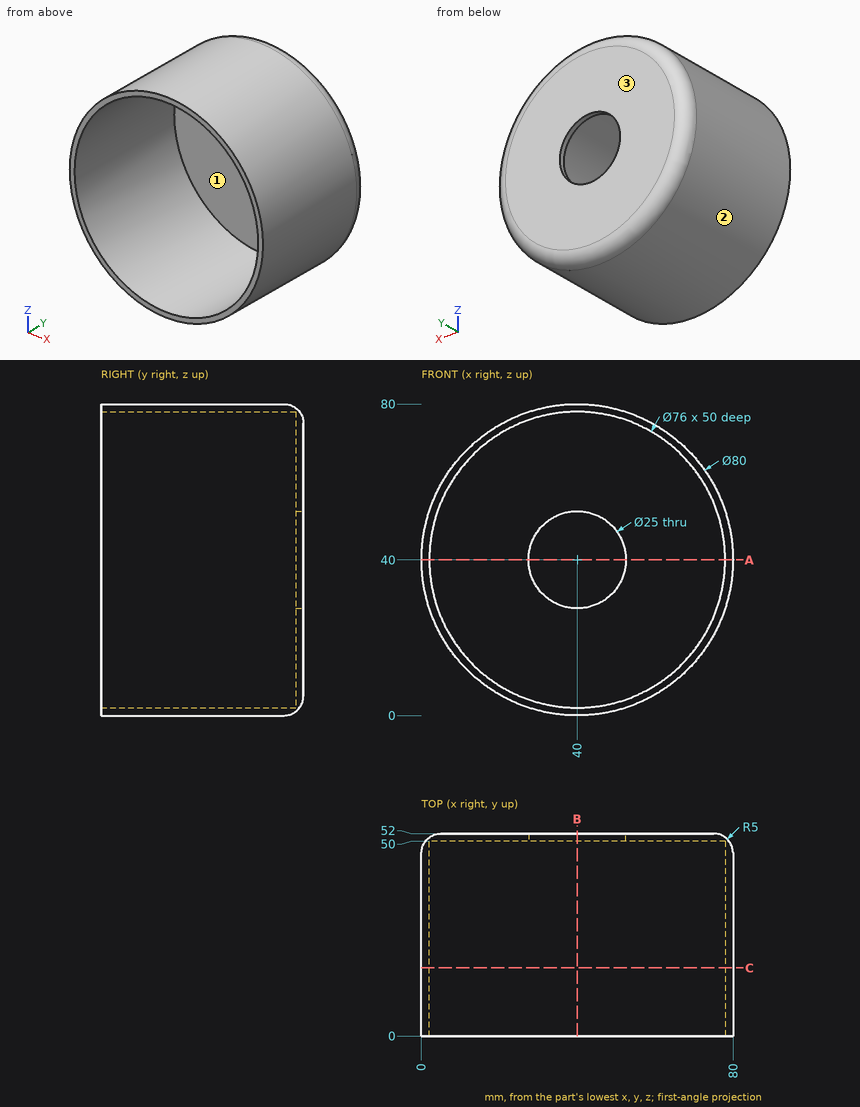
Here's the drawing with two shaded views (mm, measured from the low corner). I have some questions. Round coordinates to 2 decimals unless told otherwise and drop trailing zeros. Loops run counter-clockwise (first coordinate to the right, second up) from the corner with the lowest first, then second, coordinate; pieces in that order, holes last.
1. Will these pins go through, and if not, where does the flat tip stop? pin 1 (10 mm diameter, centred on x = 20.5, y = 13, fed in from +Z); pin 2 (12 mm diameter, centred on x = 57.5, z = 70.5, fed in from -Y); pin 3 (2 mm diameter, centred on x = 43.5, y = 41, fed in from +Z); pin 4 (3 mm diameter, centred on x = 56.5, y = 5.5, fed in from -Z).
Answers:
pin 1: stops at z = 77.28
pin 2: stops at y = 0
pin 3: stops at z = 79.92
pin 4: stops at z = 2.92
2. Suppose I cut it at C-C, the plane y = 17.5. Please give me the cut outline in (x, z), and give its area (3 significant figures).
Answers:
outline: circle Ø80 at (40, 40); hole circle Ø76 at (40, 40)
area: 490 mm2
3. If I drill on probe 1 along Z at (x, y) = (40, 51); probe 2 along Z at (x, y) = (40, 31.5); probe 3 along Y at (x, z) = (58, 48.5), over which ranges is the centre line in solid material (lowest first)?
Answers:
probe 1: z = 2 to 27.5, 52.5 to 78
probe 2: z = 0 to 2, 78 to 80
probe 3: y = 50 to 52
4. Suppose I cut it at B-B, the plane x = 40. Please give me the cut outline in (y, z), and give its area (3 significant figures).
Answers:
outline: (0, 0) - (47, 0) arc R5 ccw to (52, 5) - (52, 27.5) - (50, 27.5) - (50, 2) - (0, 2) - close; (0, 78) - (50, 78) - (50, 52.5) - (52, 52.5) - (52, 75) arc R5 ccw to (47, 80) - (0, 80) - close
area: 299 mm2
5. Thinking about a two-plate mould opening in Z: for the marked faces 1, 2 and 3, which applies, released by +Z, released by -Z, zero draft, split by the parting line, or undercut?
Answers:
face 1: undercut
face 2: split by the parting line
face 3: zero draft
6. Suppose I cut it at A-A, the plane z = 40. Please give me the cut outline in (x, y).
Answers:
outline: (0, 0) - (2, 0) - (2, 50) - (27.5, 50) - (27.5, 52) - (5, 52) arc R5 ccw to (0, 47) - close; (52.5, 50) - (78, 50) - (78, 0) - (80, 0) - (80, 47) arc R5 ccw to (75, 52) - (52.5, 52) - close
